Geometry check sheet. Reference: the model listing, model coordinates, mm. A direction names the side the tool comes from. Round coordinates to 2 decimals unless told otherwise and drop trailing zeros. Loops run counter-clockwise (first coordinate to the right, second up) from the corner with the lowest first, then second, coordinate; pieces in that order, holes last. Notation, with made-up numbers: (73.5, 5) - (91.5, 5) arc R21 cw to (91.5, 21) - close; hole circle Ø4 at (34.25, 21.5). An arc over 180 degrees is marked (long way). Write item = value, one per line.
```python
from build123d import *

# Parameters (mm, degrees)
SKETCH1_R               = 12.5
BOSS_EXTRUDE1_DEPTH     = 3
SKETCH2_W               = 3
SKETCH2_H               = 5
BOSS_EXTRUDE2_DEPTH     = 6
SKETCH3_R               = 1.5
CUT_EXTRUDE1_DEPTH      = 8.5
CUT_EXTRUDE1_DEPTH_BACK = 18.5
FILLET1_R               = 2
FILLET2_R               = 1


with BuildPart() as part:
    # Sketch1 → Boss-Extrude1 (new body)
    with BuildSketch(Plane(origin=(0, 0, 0), x_dir=(1, 0, 0), z_dir=(0, 1, 0))):
        with Locations(Location((0, 0, 0), (0, 0, 270))):  # turned: the seam where the file's is
            Circle(SKETCH1_R)
    extrude(amount=BOSS_EXTRUDE1_DEPTH)

    # Sketch2 → Boss-Extrude2 (add)
    with BuildSketch(Plane(origin=(0, 3, 0), x_dir=(1, 0, 0), z_dir=(0, 1, 0))):
        with Locations((-3.5, 0)):
            Rectangle(SKETCH2_W, SKETCH2_H)
        with Locations((3.5, 0)):
            Rectangle(SKETCH2_W, SKETCH2_H)
    extrude(amount=BOSS_EXTRUDE2_DEPTH)

    # Sketch3 → Cut-Extrude1 (cut, two sides)
    with BuildSketch(Plane(origin=(5, 0, 0), x_dir=(0, 0, -1), z_dir=(1, 0, 0))) as cut_extrude1_sk:
        with Locations((0, 7)):
            Circle(SKETCH3_R)
    extrude(amount=CUT_EXTRUDE1_DEPTH, mode=Mode.SUBTRACT)
    extrude(cut_extrude1_sk.sketch, amount=-CUT_EXTRUDE1_DEPTH_BACK, mode=Mode.SUBTRACT)

    # Fillet1
    fillet1_edges = [part.edges().sort_by_distance(p)[0] for p in [
        (3.5, 3, -2.5),
        (3.5, 3, 2.5),
        (-3.5, 3, -2.5),
        (-3.5, 3, 2.5),
    ]]
    fillet(fillet1_edges, radius=FILLET1_R)

    # Fillet2
    fillet2_edges = [part.edges().sort_by_distance(p)[0] for p in [
        (0, 0, -12.5),
    ]]
    fillet(fillet2_edges, radius=FILLET2_R)


solid = part.part
```
(1) Scan lines: L1, parallel to Y at x = 3.45, z = 0; L2, parallel to Y at x = -1, z = 5; L3, parallel to Z at x = 4.5, y = 8.25. Record each from-to range of solid material in increasing order. Write a range as [from, to].
Answers follow:
L1 = [0, 5.5], [8.5, 9]
L2 = [0, 3]
L3 = [-2.5, -0.83], [0.83, 2.5]
(2) Mould release check, pull along X, two halves, no side actions. Record for faces 1 (the flat face through (-2, 5, 0)), 2 (the flat face through (5, 5, 0)), 3 (the flat face through (-4, 7, -2.5)): pulls with the +X half, pulls with the -X half, needs draft (parallel to the pull), parting line crosses it, or undercut.
Answers follow:
face_1 = undercut
face_2 = pulls with the +X half
face_3 = needs draft
(3) Section check B-B (y = 7). Enter the section's corners in (x, z), then the cut area to 3 significant figures.
Answers follow:
outline = (-5, -2.5) - (-2, -2.5) - (-2, -1.5) - (-5, -1.5) - close; (-5, 1.5) - (-2, 1.5) - (-2, 2.5) - (-5, 2.5) - close; (2, -2.5) - (5, -2.5) - (5, -1.5) - (2, -1.5) - close; (2, 1.5) - (5, 1.5) - (5, 2.5) - (2, 2.5) - close
area = 12.0 mm²
(4) Section check A-A (z = 0). Enter the section's corners in (x, y), then the cut area to 3 significant figures.
Answers follow:
outline = (-12.5, 1) arc R1 ccw to (-11.5, 0) - (11.5, 0) arc R1 ccw to (12.5, 1) - (12.5, 3) - (5, 3) - (5, 5.5) - (2, 5.5) - (2, 3) - (-2, 3) - (-2, 5.5) - (-5, 5.5) - (-5, 3) - (-12.5, 3) - close; (-5, 8.5) - (-2, 8.5) - (-2, 9) - (-5, 9) - close; (2, 8.5) - (5, 8.5) - (5, 9) - (2, 9) - close
area = 92.6 mm²
(5) Gauge pin test, flat ends, axial feed: pin 1 (5 mm diameter, centred on y = 7, z = 0, fed in from +X); pin 2 (3.5 mm diameter, centred on x = -3.5, y = 8, fed in from -Z); pin 3 (1.8 mm diameter, centred on y = 7.5, z = 1, fed in from -X). Record the tip position at first contact, or that the pin passes through.
Answers follow:
pin_1 = 5
pin_2 = -2.5
pin_3 = -5
(6) Section check C-C (y = 4). Enter the section's corners in (x, z).
Answers follow:
outline = (-5, -2.77) - (-2, -2.77) - (-2, 2.77) - (-5, 2.77) - close; (2, -2.77) - (5, -2.77) - (5, 2.77) - (2, 2.77) - close
(7) Set-up check for faces 4 (the flat face through (2, 5, 0)), 5 (the flat face through (-4, 7, 2.5)), 6 (the flat face through (3, 7, -2.5)), 7 (the flat face through (-5, 5, 0)): record each of +Z, -Z, +X, -X, +Y, -Y from which the full face is reachable in a straight line by a thin tool's end or side.
Answers follow:
face_4 = +Z, -Z, +Y
face_5 = +Z, +X, -X, +Y
face_6 = -Z, +X, -X, +Y
face_7 = +Z, -Z, -X, +Y
(8) Section check D-D (x = 0). Enter the section's corners in (y, z), then the cut area to 3 significant figures.
Answers follow:
outline = (0, -11.5) arc R1 ccw to (1, -12.5) - (3, -12.5) - (3, 12.5) - (1, 12.5) arc R1 ccw to (0, 11.5) - close
area = 74.6 mm²
